Build history of the part. All positions in model axes, mm. Face numbers are marked on the shaded views. Give positions to 0.01 mm unless a question says otherwise; leave off trailing zeros. Loops run counter-clockwise (first coordinate to the right, second up) from the corner with the lowest first, then second, coordinate; pieces in that order, holes last. Notation, with made-up numbers: M 11,-34.75 L 15,-34.75 A7 ccw 15,-24.75 Z; hole C -10.75,17.25 d2. An arc over 180 degrees is marked long. Answer as a JSON object with one key per item and string values. Group by question number.
1. Drill centre lines: line 1 along Z through (x, y) = (-1.45, 356) (3 decimals); line 2 along Z through (x, y) = (-11.75, 356); line 3 along Z through (x, y) = (-5.25, 76.5). Where is each one in solid material? Low to high. Write a range as [from, to].
2. Mould opens along X. For the marked faces 1, 2 and 3 say: released by +X, released by -X, zero draft, split by the parting line, or undercut.
3. Slice it at A-A (y = 234.5). List the corners of the cut face in (x, z).
4. Drop flat-ended pins along their axis: pin 1 Ø6.5 at (y, z) = (355.5, 31.5) entering from +X; pin 2 Ø0.8 at (x, z) = (-8.5, 54) entering from +Y; pin 3 Ø11 at (y, z) = (356, 28.5) entering from +X. Give the stop position or say it passes through.
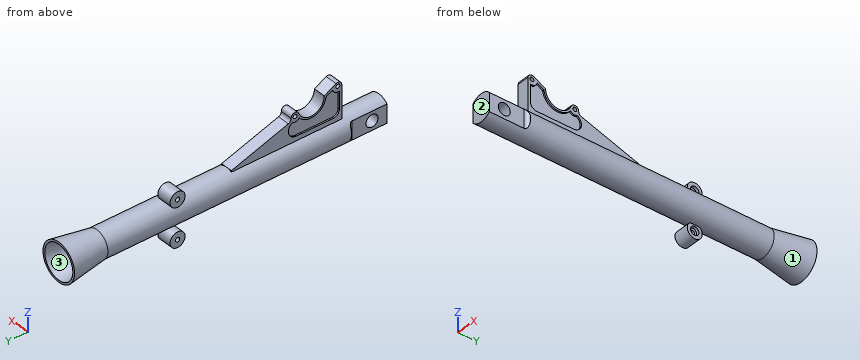
from build123d import *

# Parameters (mm, degrees)
SKETCH1_R                = 22.5
BOSS_EXTRUDE1_DEPTH      = 470
SKETCH2_R                = 32
CUT_EXTRUDE1_DEPTH       = 536.415959904
HOLE1_START              = -16.5
HOLE1_OUTLINE_R          = 10
HOLE1_DEPTH              = 33
SKETCH5_R                = 12.5
BOSS_EXTRUDE2_DEPTH      = 25
BOSS_EXTRUDE3_REACH      = 553.123
BOSS_EXTRUDE3_END_RADIUS = 22.5
SKETCH8_W                = 20
SKETCH8_H                = 184
CUT_EXTRUDE2_DEPTH       = 543.665873365
SKETCH11_R               = 3.25
CUT_EXTRUDE3_DEPTH       = 542.321069343
CUT_EXTRUDE4_DEPTH       = 2.5


# Read off the part's stored shape, not the designer's step: Shell1, Hole1
with BuildPart() as part:
    # Sketch1 → Boss-Extrude1 (new body)
    with BuildSketch(Plane(origin=(0, 0, 0), x_dir=(1, 0, 0), z_dir=(0, 1, 0))):
        with Locations(Location((0, 0, 0), (0, 0, 90))):
            Circle(SKETCH1_R)
    extrude(amount=BOSS_EXTRUDE1_DEPTH)

    # Sketch2 → section 0 of loft1
    with BuildSketch(Plane(origin=(0, 533.5, 0), x_dir=(1, 0, 0), z_dir=(0, 1, 0)), mode=Mode.PRIVATE) as loft1_s0:
        Circle(SKETCH2_R)
    # loft up to a face of the part (loft1)
    loft([loft1_s0.sketch, Face(Wire([part.edges().sort_by_distance((-16.401794117, 470, 15.402309883))[0]]))])

    # Shell1 outline → Shell1 (revolve, cut)
    with BuildSketch(Plane.XY):
        Polygon((28.461048171, 533.5), (0, 533.5), (0, 67), (19, 67), (19, 470.260362226), align=None)
    revolve(axis=Axis((0, 0, 0), (0, 1, 0)), mode=Mode.SUBTRACT)

    # Sketch3 → Cut-Extrude1 (cut, symmetric)
    with BuildSketch(Plane.XY):
        with BuildLine():
            Line((22.5, 64), (44.504485309, 64))
            Line((44.504485309, 64), (44.504485309, -12.1793828))
            Line((44.504485309, -12.1793828), (16.5, -12.1793828))
            Line((16.5, -12.1793828), (16.5, 58))
            ThreePointArc((16.5, 58), (18.257359313, 62.242640687), (22.5, 64))
        make_face()
    cut_extrude1 = extrude(amount=CUT_EXTRUDE1_DEPTH, both=True, mode=Mode.SUBTRACT)

    # Mirror1: Cut-Extrude1 across plane
    add(cut_extrude1.mirror(Plane(origin=(0, 0, 0), x_dir=(0, 0, 1), z_dir=(1, 0, 0))), mode=Mode.SUBTRACT)

    # Hole1 outline → Hole1 (cut)
    with BuildSketch(Plane.YZ.offset(HOLE1_START)):
        with Locations((25, 0)):
            Circle(HOLE1_OUTLINE_R)
    extrude(amount=HOLE1_DEPTH, mode=Mode.SUBTRACT)

    # Sketch5 → Boss-Extrude2 (add)
    with BuildSketch(Plane(origin=(0, 0, 0), x_dir=(0, 0, -1), z_dir=(1, 0, 0))):
        with Locations((-32, 356)):
            Circle(SKETCH5_R)
    boss_extrude2 = extrude(amount=-BOSS_EXTRUDE2_DEPTH)

    # Sketch7 → CBORE for M6 Hex Head Machine Screw1 (revolve, cut)
    with BuildSketch(Plane(origin=(0, 356, 32), x_dir=(0, 0, -1), z_dir=(0, 1, 0))):
        Polygon((0, 0), (0, 32.0001), (3.5, 32.0001), (3.5, 4.7), (6.975, 4.7), (6.975, 0.025), (7, 0), align=None)
    cbore_for_m6_hex_head_machine_screw1 = revolve(axis=Axis((6.35, 356, 32), (-1, 0, 0)), mode=Mode.SUBTRACT)

    # Mirror2: Boss-Extrude2, CBORE for M6 Hex Head Machine Screw1 across plane
    add(boss_extrude2.mirror(Plane.XY))
    add(cbore_for_m6_hex_head_machine_screw1.mirror(Plane.XY), mode=Mode.SUBTRACT)

    # Boss-Extrude3: up to this cylinder (the profile starts outside it)
    boss_extrude3_end = Plane(origin=(0, 162, 0), z_dir=(0, -1, 0)) * Cylinder(BOSS_EXTRUDE3_END_RADIUS, 1152.246, mode=Mode.PRIVATE)
    # Sketch8 → Boss-Extrude3 (add, up to the surface)
    with BuildSketch(Plane.XY.offset(90), mode=Mode.PRIVATE) as boss_extrude3_sk1:
        with Locations((0, 162)):
            Rectangle(SKETCH8_W, SKETCH8_H)
    boss_extrude3_tool1 = extrude(boss_extrude3_sk1.sketch, amount=-BOSS_EXTRUDE3_REACH, mode=Mode.PRIVATE) - boss_extrude3_end
    add(boss_extrude3_tool1.solids().sort_by_distance((0, 162, 90))[0])

    # Sketch10 → Cut-Extrude2 (cut, through all)
    with BuildSketch(Plane(origin=(10, 0, 0), x_dir=(0, 0, -1), z_dir=(1, 0, 0))):
        with BuildLine():
            Line((-90, 70), (-90, 254))
            Line((-90, 254), (-22.5, 254))
            Line((-22.5, 254), (-53.39120023, 158.926661609))
            ThreePointArc((-53.39120023, 158.926661609), (-55.83933924, 155.614626187), (-59.786533793, 154.438778235))
            ThreePointArc((-59.786533793, 154.438778235), (-66.375955373, 149.206085442), (-62.280701754, 141.855544753))
            ThreePointArc((-62.280701754, 141.855544753), (-48.37626649, 117.202834204), (-70.262213343, 99.255834796))
            Line((-70.262213343, 99.255834796), (-80.739159354, 79.551565158))
            ThreePointArc((-80.739159354, 79.551565158), (-80.571587455, 73.152252513), (-75, 70))
            Line((-75, 70), (-90, 70))
        make_face()
    extrude(amount=-CUT_EXTRUDE2_DEPTH, mode=Mode.SUBTRACT)

    # Sketch11 → Cut-Extrude3 (cut, through all)
    with BuildSketch(Plane(origin=(10, 0, 0), x_dir=(0, 0, -1), z_dir=(1, 0, 0))):
        with Locations(Location((-60, 147.942284398, 0), (0, 0, 90))):
            Circle(SKETCH11_R)
        with Locations(Location((-75, 76.5, 0), (0, 0, 90))):
            Circle(SKETCH11_R)
    extrude(amount=-CUT_EXTRUDE3_DEPTH, mode=Mode.SUBTRACT)

    # Sketch12 → Cut-Extrude4 (cut)
    with BuildSketch(Plane(origin=(10, 0, 0), x_dir=(0, 0, -1), z_dir=(1, 0, 0))):
        with BuildLine():
            Line((-27.655644371, 146), (-27.655644371, 84))
            ThreePointArc((-27.655644371, 84), (-30.584576559, 76.928932188), (-37.655644371, 74))
            Line((-37.655644371, 74), (-66.354191767, 74))
            ThreePointArc((-66.354191767, 74), (-67.285494294, 81.135342674), (-73.14840788, 85.307474475))
            Line((-73.14840788, 85.307474475), (-67.247053013, 96.406308753))
            ThreePointArc((-67.247053013, 96.406308753), (-45.973818024, 114.344671566), (-54.467499716, 140.843591518))
            ThreePointArc((-54.467499716, 140.843591518), (-51.192765452, 146.089551388), (-52.076348436, 152.210275248))
            ThreePointArc((-52.076348436, 152.210275248), (-37.4516744, 158.598991088), (-27.655644371, 146))
        make_face()
    cut_extrude4 = extrude(amount=-CUT_EXTRUDE4_DEPTH, mode=Mode.SUBTRACT)

    # Mirror3: Cut-Extrude4 across plane
    add(cut_extrude4.mirror(Plane(origin=(0, 0, 0), x_dir=(0, 0, 1), z_dir=(1, 0, 0))), mode=Mode.SUBTRACT)


solid = part.part
Established:
{
 "1": {"line 1": "z = [-44.5, -38.975], [-25.025, -18.945], [18.945, 25.025], [38.975, 44.5]", "line 2": "z = [-44.5, -35.5], [-28.5, -19.5], [-19.19, -14.93], [14.93, 19.19], [19.5, 28.5], [35.5, 44.5]", "line 3": "z = [-21.88, -18.26], [18.26, 71.75], [78.25, 81.5]"},
 "2": {"face 1": "split by the parting line", "face 2": "zero draft", "face 3": "undercut"},
 "3": {"outline": "M -10,20.16 A22.5 ccw long 10,20.16 L 10,28.84 L -10,28.84 Z; hole C 0,0 d38"},
 "4": {"pin 1": "stops at x = -4.7", "pin 2": "stops at y = 158.37", "pin 3": "stops at x = 0"}
}
